```python
from build123d import *

# Parameters (mm, degrees)
SCHIZZO1_W                   = 15.3
SCHIZZO1_H                   = 12.5
ESTRUSIONE_ESTRUSIONE1_DEPTH = 6
SCHIZZO2_W                   = 1.5
SCHIZZO2_H                   = 1.25
TAGLIO_ESTRUSIONE1_DEPTH     = 19.055470085
SCHIZZO3_W                   = 10.85
SCHIZZO3_H                   = 12.85
TAGLIO_ESTRUSIONE2_DEPTH     = 19.055470085
SCHIZZO4_W                   = 6.5
SCHIZZO4_H                   = 2.3
TAGLIO_ESTRUSIONE3_DEPTH     = 19.055470085
SCHIZZO5_W                   = 1.5
SCHIZZO5_H                   = 7.75
TAGLIO_ESTRUSIONE4_DEPTH     = 19.055470085
ESTRUSIONE_ESTRUSIONE2_REACH = 22.139
SCHIZZO6_R                   = 3
SCHIZZO7_W                   = 4
SCHIZZO7_H                   = 4
ESTRUSIONE_ESTRUSIONE3_DEPTH = 0.4
SMUSSO1_SIZE                 = 0.5
SMUSSO2_SIZE                 = 0.5
SMUSSO3_SIZE                 = 0.5
SMUSSO4_SIZE                 = 0.5
RACCORDO1_R                  = 4.35
RACCORDO2_R                  = 4.5


with BuildPart() as part:
    # Schizzo1 → Estrusione-Estrusione1 (new body)
    with BuildSketch(Plane(origin=(-3, 0, 0), x_dir=(0, -1, 0), z_dir=(-1, 0, 0))):
        with Locations((-5.35, -4.75)):
            Rectangle(SCHIZZO1_W, SCHIZZO1_H)
    extrude(amount=-ESTRUSIONE_ESTRUSIONE1_DEPTH)

    # Schizzo2 → Taglio-Estrusione1 (cut, through all)
    with BuildSketch(Plane(origin=(3, 0, 0), x_dir=(0, 0, -1), z_dir=(1, 0, 0))):
        with Locations((-0.75, 12.375)):
            Rectangle(SCHIZZO2_W, SCHIZZO2_H)
    extrude(amount=-TAGLIO_ESTRUSIONE1_DEPTH, mode=Mode.SUBTRACT)

    # Schizzo3 → Taglio-Estrusione2 (cut, through all)
    with BuildSketch(Plane(origin=(3, 0, 0), x_dir=(0, 0, -1), z_dir=(1, 0, 0))):
        with Locations((5.575, 6.575)):
            Rectangle(SCHIZZO3_W, SCHIZZO3_H)
    extrude(amount=-TAGLIO_ESTRUSIONE2_DEPTH, mode=Mode.SUBTRACT)

    # Schizzo4 → Taglio-Estrusione3 (cut, through all)
    with BuildSketch(Plane(origin=(3, 0, 0), x_dir=(0, 0, -1), z_dir=(1, 0, 0))):
        with Locations((1.75, -1.15)):
            Rectangle(SCHIZZO4_W, SCHIZZO4_H)
    extrude(amount=-TAGLIO_ESTRUSIONE3_DEPTH, mode=Mode.SUBTRACT)

    # Schizzo5 → Taglio-Estrusione4 (cut, through all)
    with BuildSketch(Plane(origin=(3, 0, 0), x_dir=(0, 0, -1), z_dir=(1, 0, 0))):
        with Locations((-0.75, 3.875)):
            Rectangle(SCHIZZO5_W, SCHIZZO5_H)
    extrude(amount=-TAGLIO_ESTRUSIONE4_DEPTH, mode=Mode.SUBTRACT)

    # Schizzo6 → Estrusione-Estrusione2 (add, up to next)
    with BuildSketch(Plane.XZ.offset(3.6), mode=Mode.PRIVATE) as estrusione_estrusione2_sk1:
        with Locations(Location((0, -8, 0), (0, 0, 90))):
            Circle(SCHIZZO6_R)
    estrusione_estrusione2_tool1 = extrude(estrusione_estrusione2_sk1.sketch, amount=-ESTRUSIONE_ESTRUSIONE2_REACH, mode=Mode.PRIVATE) - part.part
    add(estrusione_estrusione2_tool1.solids().sort_by_distance((0, -3.6, -8))[0])

    # Schizzo7 → Estrusione-Estrusione3 (add)
    with BuildSketch(Plane.XZ.offset(3.6)):
        with Locations((0, -8)):
            Rectangle(SCHIZZO7_W, SCHIZZO7_H)
    extrude(amount=ESTRUSIONE_ESTRUSIONE3_DEPTH)

    # Smusso1
    smusso1_edges = [part.edges().sort_by_distance(p)[0] for p in [
        (-2, -3.8, -10),
    ]]
    chamfer(smusso1_edges, length=SMUSSO1_SIZE)

    # Smusso2
    smusso2_edges = [part.edges().sort_by_distance(p)[0] for p in [
        (2, -3.8, -6),
    ]]
    chamfer(smusso2_edges, length=SMUSSO2_SIZE)

    # Smusso3
    smusso3_edges = [part.edges().sort_by_distance(p)[0] for p in [
        (-2, -3.8, -6),
    ]]
    chamfer(smusso3_edges, length=SMUSSO3_SIZE)

    # Smusso4
    smusso4_edges = [part.edges().sort_by_distance(p)[0] for p in [
        (2, -3.8, -10),
    ]]
    chamfer(smusso4_edges, length=SMUSSO4_SIZE)

    # Raccordo1
    raccordo1_edges = [part.edges().sort_by_distance(p)[0] for p in [
        (0, 0.15, -0.15),
    ]]
    fillet(raccordo1_edges, radius=RACCORDO1_R)

    # Raccordo2
    raccordo2_edges = [part.edges().sort_by_distance(p)[0] for p in [
        (0, 0, 0),
    ]]
    fillet(raccordo2_edges, radius=RACCORDO2_R)


solid = part.part
```
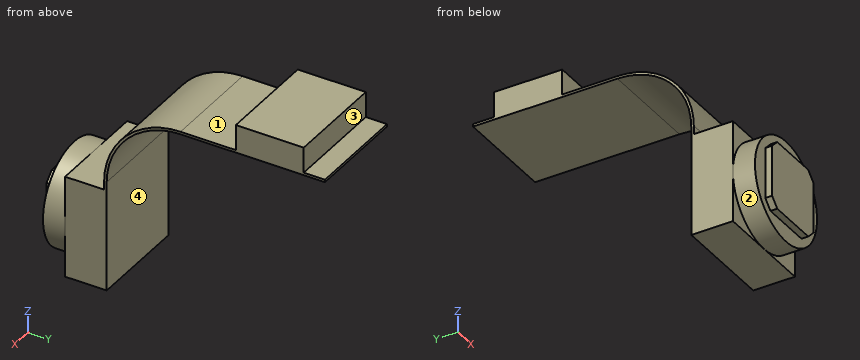
Geometry: final body of the model. Coordinates: model frame, mm. Face numbers are marked on the shaded views. A direction names the side the tool comes from. Coordinates: 2 decimals unless noted, no trailing zeros. Write each loop counter-clockwise with the first axis right and the second up, starting at its lowest first coordinate (ties: lowest second). Pieces come first, ordered by that corner, then holes. Notation, with made-up numbers: M -22,-11.75 L 34,-11.75 A16 cw 34,-2.75 Z; hole C 30,81.25 d6. An arc over 180 degrees is marked long. Answer as CSV lines item,"result". Start each with the question number.
Q1. Cut plane A-A on x = -1. Return the cut outline in (y, z).
Q2. Line query: line 1 (Z direction, x = -0.75, y = -1.5); line 2 (Y direction, x = -1.75, z = -8.25); line 3 (Y direction, x = 0.05, z = -5.25). Output: solid intervals per line, ascending. Write a range as from..to.
Q3. Pin query (flat end, axial travel): P1, Ø2, axis at x = 1, z = -9, coming from the +Y side; P2, Ø1.5, axis at x = -2.5, z = -6, coming from the +Y side; P3, Ø2.5, axis at x = -0.5, y = -1.5, coming from the +Z side. Return the tip coordinate at first contact, or that it passes through.
Q4. Cut plane D-D on x = -2.6. Return the cut outline in (y, z).
Q5. Cut plane B-B on z = -6.25. Return the cut outline in (x, y).
Q6. Reachability of the marked faces 1, 2, 3 and 4 from +Z, -Z, +X, -X, +Y, -Y: full face, straight path, thin tool, end or side. Return the list, or none.
Q7. Cut plane C-C on y = 4.75. Return the cut outline in (x, z), then the cut area to 3 significant figures.
Findings below:
1,outline,"M -4,-10 L -3.6,-10 L -3.6,-10.83 L -2.3,-10.83 L -2.3,-11 L 0.15,-11 L 0.15,-4.5 A4.35 cw 4.5,-0.15 L 13,-0.15 L 13,0 L 11.75,0 L 11.75,1.5 L 7.75,1.5 L 7.75,0 L 4.5,0 A4.5 ccw 0,-4.5 L 0,-5 L -2.3,-5 L -2.3,-5.17 L -3.6,-5.17 L -3.6,-6 L -4,-6 Z"
2,line 1,"z = -11..-5"
2,line 2,"y = -4..0.15"
2,line 3,"y = -3.6..0.15"
3,P1,"stops at y = 0.15"
3,P2,"stops at y = 0.15"
3,P3,"stops at z = -5"
4,outline,"M -3.6,-9.5 L -2.3,-9.5 L -2.3,-11 L 0.15,-11 L 0.15,-4.5 A4.35 cw 4.5,-0.15 L 13,-0.15 L 13,0 L 11.75,0 L 11.75,1.5 L 7.75,1.5 L 7.75,0 L 4.5,0 A4.5 ccw 0,-4.5 L 0,-5 L -2.3,-5 L -2.3,-6.5 L -3.6,-6.5 Z"
5,outline,"M -3,-2.3 L -2.44,-2.3 L -2.44,-3.6 L -1.75,-3.6 L -1.75,-4 L 1.75,-4 L 1.75,-3.6 L 2.44,-3.6 L 2.44,-2.3 L 3,-2.3 L 3,0.15 L -3,0.15 Z"
6,face 1,"+Z, +X, -X, -Y"
6,face 2,"-Y"
6,face 3,"+Z, +X, -X, +Y"
6,face 4,"-Z, +X, -X, +Y"
7,outline,"M -3,-0.15 L 3,-0.15 L 3,0 L -3,0 Z"
7,area,"0.900 mm2"
